Here's how the part is built. I have some questions about the finished solid (model axes, mm). Coordinates: 2 decimals unless noted, no trailing zeros. Write each loop counter-clockwise with the first axis right and the second up, starting at its lowest first coordinate (ties: lowest second). Pieces come first, ordered by that corner, then holes. Notation, with made-up numbers: (51.25, 80) - (68.25, 80) arc R10 cw to (68.25, 84) - close; hole circle Ø2 at (6.25, 67). An arc over 180 degrees is marked (long way). Answer in a Markdown table with one row per item. Add a question column.
Item 1: I'm going to push flat-ended pins straight in: pin 1 (6 mm diameter, centred on x = -107.5, z = 5.5, fed in from -Y); pin 2 (12 mm diameter, centred on x = 136.5, z = -8, fed in from +Y); pin 3 (5 mm diameter, centred on y = 154, z = -7, fed in from +X); pin 4 (12 mm diameter, centred on y = 201.5, z = -9, fed in from -X). Where does each tip first touch, or does it pass through?
Item 2: Imagine slicing it at B-B (x = -14.5). Please give me the cut outline in (y, z).
Item 3: If I drill on probe 1 along X at (y, z) = (296.5, 8); probe 2 along Z at (x, y) = (90, 407); probe 3 along Z at (x, y) = (-115, 176), over which ranges is the centre line in solid material (lowest first)? Write a range as from..to.
Item 4: Imagine slicing it at A-A (y = 162). Please give me the cut outline in (x, z), plus the area to 3 significant figures.
Item 5: Imagine slicing it at C-C (x = 192). Please give me the cut outline in (y, z), plus the area to 3 significant figures.
from build123d import *

# Parameters (mm, degrees)
THICKEN1_DEPTH     = 442
THICKEN1_2_DEPTH   = 251.51
THICKEN1_START     = 279.51
THICKEN1_3_DEPTH   = 162.49
SKETCH4_R          = 5
CUT_EXTRUDE1_DEPTH = 20
SKETCH5_R          = 5
CUT_EXTRUDE2_DEPTH = 20
CUT_EXTRUDE3_START = -20
SKETCH7_R          = 5
CUT_EXTRUDE3_DEPTH = 20


# Read off the part's stored shape, not the designer's step: Thicken1
with BuildPart() as part:
    # Thicken1 outline → Thicken1 (new body)
    with BuildSketch(Plane(origin=(0, 0, 0), x_dir=(1, 0, 0), z_dir=(0, 1, 0))):
        with BuildLine():
            ThreePointArc((-234.724558603, 8.605268641), (0, -2.4), (234.724558603, 8.605268641))
            Line((234.724558603, 8.605268641), (234.275441397, 13.384211383))
            ThreePointArc((234.275441397, 13.384211383), (0, 2.4), (-234.275441397, 13.384211383))
            Line((-234.275441397, 13.384211383), (-234.724558603, 8.605268641))
        make_face()
    extrude(amount=THICKEN1_DEPTH)

    # Thicken1 2 outline → Thicken1 2 (add)
    with BuildSketch(Plane(origin=(0, 0, 0), x_dir=(1, 0, 0), z_dir=(0, 1, 0))):
        with BuildLine():
            Line((234.275441397, 13.384211383), (234.724558603, 8.605268641))
            ThreePointArc((234.724558603, 8.605268641), (242.420228217, 9.340459098), (250.113595715, 10.099361169))
            ThreePointArc((250.113595715, 10.099361169), (257.181828344, 7.101502773), (260.1, 0))
            Line((260.1, 0), (260.1, -16))
            Line((260.1, -16), (264.9, -16))
            Line((264.9, -16), (264.9, 0))
            ThreePointArc((264.9, 0), (260.491504347, 10.580091518), (249.874719929, 14.89947331))
            ThreePointArc((249.874719929, 14.89947331), (242.076266252, 14.129636973), (234.275441397, 13.384211383))
        make_face()
        with BuildLine():
            ThreePointArc((-250.113595715, 10.099361169), (-242.420228217, 9.340459098), (-234.724558603, 8.605268641))
            Line((-234.724558603, 8.605268641), (-234.275441397, 13.384211383))
            ThreePointArc((-234.275441397, 13.384211383), (-242.076266252, 14.129636973), (-249.874719929, 14.89947331))
            ThreePointArc((-249.874719929, 14.89947331), (-260.491504347, 10.580091518), (-264.9, 0))
            Line((-264.9, 0), (-264.9, -16))
            Line((-264.9, -16), (-260.1, -16))
            Line((-260.1, -16), (-260.1, 0))
            ThreePointArc((-260.1, 0), (-257.181828344, 7.101502773), (-250.113595715, 10.099361169))
        make_face()
    extrude(amount=THICKEN1_2_DEPTH)

    # Thicken1 3 outline → Thicken1 3 (add)
    with BuildSketch(Plane(origin=(0, 0, 0), x_dir=(1, 0, 0), z_dir=(0, 1, 0)).offset(THICKEN1_START)):
        with BuildLine():
            Line((234.275441397, 13.384211383), (234.724558603, 8.605268641))
            ThreePointArc((234.724558603, 8.605268641), (242.420228217, 9.340459098), (250.113595715, 10.099361169))
            ThreePointArc((250.113595715, 10.099361169), (257.181828344, 7.101502773), (260.1, 0))
            Line((260.1, 0), (260.1, -16))
            Line((260.1, -16), (264.9, -16))
            Line((264.9, -16), (264.9, 0))
            ThreePointArc((264.9, 0), (260.491504347, 10.580091518), (249.874719929, 14.89947331))
            ThreePointArc((249.874719929, 14.89947331), (242.076266252, 14.129636973), (234.275441397, 13.384211383))
        make_face()
        with BuildLine():
            ThreePointArc((-250.113595715, 10.099361169), (-242.420228217, 9.340459098), (-234.724558603, 8.605268641))
            Line((-234.724558603, 8.605268641), (-234.275441397, 13.384211383))
            ThreePointArc((-234.275441397, 13.384211383), (-242.076266252, 14.129636973), (-249.874719929, 14.89947331))
            ThreePointArc((-249.874719929, 14.89947331), (-260.491504347, 10.580091518), (-264.9, 0))
            Line((-264.9, 0), (-264.9, -16))
            Line((-264.9, -16), (-260.1, -16))
            Line((-260.1, -16), (-260.1, 0))
            ThreePointArc((-260.1, 0), (-257.181828344, 7.101502773), (-250.113595715, 10.099361169))
        make_face()
    extrude(amount=THICKEN1_3_DEPTH)

    # Sketch4 → Cut-Extrude1 (cut)
    with BuildSketch(Plane(origin=(250, 0, 0), x_dir=(0, 0, -1), z_dir=(1, 0, 0))):
        with Locations(Location((0, 346.755, 0), (0, 0, 90))):
            Circle(SKETCH4_R)
    extrude(amount=CUT_EXTRUDE1_DEPTH, mode=Mode.SUBTRACT)

    # Sketch5 → Cut-Extrude2 (cut)
    with BuildSketch(Plane(origin=(250, 0, 0), x_dir=(0, 0, -1), z_dir=(1, 0, 0))):
        with Locations(Location((0, 125.755, 0), (0, 0, 270))):
            Circle(SKETCH5_R)
    extrude(amount=CUT_EXTRUDE2_DEPTH, mode=Mode.SUBTRACT)

    # Sketch7 → Cut-Extrude3 (cut)
    with BuildSketch(Plane(origin=(-250, 0, 0), x_dir=(0, 0, -1), z_dir=(1, 0, 0)).offset(CUT_EXTRUDE3_START)):
        with Locations(Location((0, 346.755, 0), (0, 0, 90))):
            Circle(SKETCH7_R)
        with Locations(Location((0, 125.755, 0), (0, 0, 270))):
            Circle(SKETCH7_R)
    extrude(amount=CUT_EXTRUDE3_DEPTH, mode=Mode.SUBTRACT)


solid = part.part
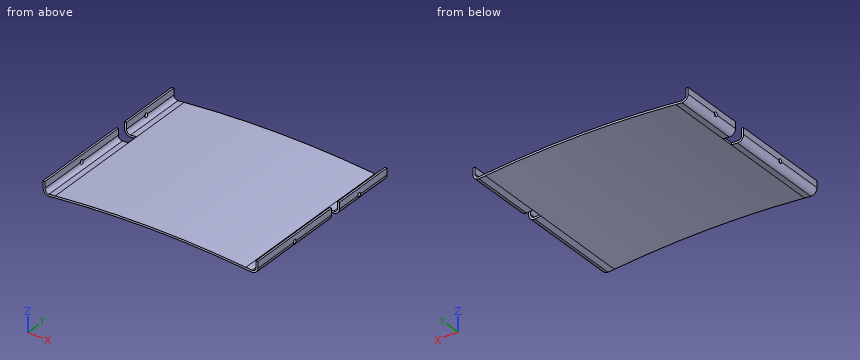
Here are the results:
| question | item | result |
|---|---|---|
| 1 | pin 1 | passes through |
| 1 | pin 2 | stops at y = 442 |
| 1 | pin 3 | stops at x = 264.2 |
| 1 | pin 4 | stops at x = -264.59 |
| 2 | outline | (0, -2.44) - (442, -2.44) - (442, 2.36) - (0, 2.36) - close |
| 3 | probe 1 | x = -264.9..-260.1, 260.1..264.9 |
| 3 | probe 2 | z = -4.02..0.79 |
| 3 | probe 3 | z = -5.04..-0.24 |
| 4 | outline | (-264.9, 0) arc R14.9 ccw to (-249.87, -14.9) arc R2503.85 cw to (-234.28, -13.38) arc R2503.85 cw to (234.28, -13.38) arc R2503.85 cw to (249.87, -14.9) arc R14.9 ccw to (264.9, 0) - (264.9, 16) - (260.1, 16) - (260.1, 0) arc R10.1 cw to (250.11, -10.1) arc R2508.65 ccw to (234.72, -8.61) arc R2508.65 ccw to (-234.72, -8.61) arc R2508.65 ccw to (-250.11, -10.1) arc R10.1 cw to (-260.1, 0) - (-260.1, 16) - (-264.9, 16) - close |
| 4 | area | 2,750 mm2 |
| 5 | outline | (0, -9.77) - (442, -9.77) - (442, -4.96) - (0, -4.96) - close |
| 5 | area | 2,130 mm2 |
